Model file for the job. Use its own axes, mm. Face numbers are marked on the shaded views. A direction names the side the tool comes from. Give positions to 0.01 mm unless a question says otherwise; leave off trailing zeros. Write each loop counter-clockwise with the first axis right and the second up, starting at its lowest first coordinate (ties: lowest second). Pieces come first, ordered by that corner, then holes. Notation, with made-up numbers: (28, 67.5) - (67, 67.5) arc R14 cw to (67, 93.5) - close; hole circle Ø9 at (43.25, -29.5). An arc over 180 degrees is marked (long way). Use a Markdown table: item, result. Add a question column.
```python
from build123d import *

# Parameters (mm, degrees)
F2_DEPTH = 35


with BuildPart() as f2:
    # F1 (on Top) + F0 (on Top) → F2 (new body)
    with BuildSketch(Plane.XY):
        Polygon((-16.83088, -2.557084), (0, -2.557084), (0, 0), (-14.142136, 14.142136), (-12.975409, 15.308862), (-10.107344, 12.440796), (-8.69313, 13.85501), (-12.823902, 17.985781), (-14.238115, 16.571568), (-16.83088, 14.142136), align=None)
        Polygon((-14.142136, 11.453391), (-2.688745, 0), (-14.142136, 0), align=None, mode=Mode.SUBTRACT)
    with BuildSketch(Plane.XY):
        Polygon((14.142136, 14.142136), (0, 0), (0, -2.557084), (16.83088, -2.557084), (16.83088, 14.142136), (14.238115, 16.571568), (12.823902, 17.985781), (8.69313, 13.85501), (10.107344, 12.440796), (12.975409, 15.308862), align=None)
        Polygon((2.688745, 0), (14.142136, 11.453391), (14.142136, 0), align=None, mode=Mode.SUBTRACT)
    extrude(amount=F2_DEPTH)


solid = f2.part
```
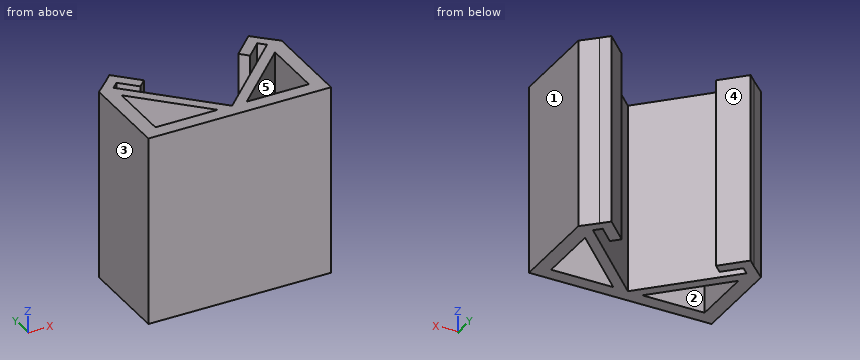
(1) Band-saw the part on C-C (y = 9). Write the cut outline in (x, z).
(2) Band-saw the part on D-D (y = 14.75). Write the cut outline in (x, z).
(3) Probe probe 1 along X at (y, z) = (10, 27); probe 2 along X at (y, z) = (1, 32.5); probe 3 along Y at (x, z) = (13, 11). List the from-to ranges inside material, lowest first. Write a range as [from, to].
(4) Band-saw the part on A-A (z = 11). Write the cut outline in (x, y) (3 decimals).
(5) Two-plate mould, pull along Y, no slides. Class the marked faces 3, 4 and 5: +Y half, -Y half, draft (parallel to the pull), parting line (faces both ways), or undercut.
(6) Which spindle directions (+Z, -Z, +X, -X, +Y, -Y) get a long thin tool onto all of the face, cutting with end or side? Do the marked faces 1 and 2. Say none if no direction does.
(7) Flat gauge pins, fed straight in: pin 1 (1.5 mm diameter, centred on x = 10, y = 2, fed in from +Z); pin 2 (2 mm diameter, centred on x = -11, z = 26.5, fed in from +Y). Where does each tip first touch, or does it go through?
(8) Band-saw the part on B-B (x = -5.5). Write the cut outline in (y, z).
Model answer:
| question | item | result |
|---|---|---|
| 1 | outline | (-16.83, 0) - (-14.14, 0) - (-14.14, 35) - (-16.83, 35) - close; (-11.69, 0) - (-9, 0) - (-9, 35) - (-11.69, 35) - close; (9, 0) - (11.69, 0) - (11.69, 35) - (9, 35) - close; (14.14, 0) - (16.83, 0) - (16.83, 35) - (14.14, 35) - close |
| 2 | outline | (-16.18, 0) - (-13.53, 0) - (-13.53, 35) - (-16.18, 35) - close; (-12.42, 0) - (-9.59, 0) - (-9.59, 35) - (-12.42, 35) - close; (9.59, 0) - (12.42, 0) - (12.42, 35) - (9.59, 35) - close; (13.53, 0) - (16.18, 0) - (16.18, 35) - (13.53, 35) - close |
| 3 | probe 1 | x = [-16.83, -14.14], [-12.69, -10], [10, 12.69], [14.14, 16.83] |
| 3 | probe 2 | x = [-16.83, -14.14], [-3.69, -1], [1, 3.69], [14.14, 16.83] |
| 3 | probe 3 | y = [-2.56, 0], [10.31, 13], [15.28, 17.81] |
| 4 | outline | (-16.831, -2.557) - (16.831, -2.557) - (16.831, 14.142) - (14.238, 16.572) - (12.824, 17.986) - (8.693, 13.855) - (10.107, 12.441) - (12.975, 15.309) - (14.142, 14.142) - (0, 0) - (-14.142, 14.142) - (-12.975, 15.309) - (-10.107, 12.441) - (-8.693, 13.855) - (-12.824, 17.986) - (-14.238, 16.572) - (-16.831, 14.142) - close; hole (-14.142, 0) - (-2.689, 0) - (-14.142, 11.453) - close; hole (2.689, 0) - (14.142, 0) - (14.142, 11.453) - close |
| 5 | face 3 | draft |
| 5 | face 4 | +Y half |
| 5 | face 5 | undercut |
| 6 | face 1 | +Z, -Z, +X, +Y, -Y |
| 6 | face 2 | +Z, -Z |
| 7 | pin 1 | passes through |
| 7 | pin 2 | stops at y = 17.16 |
| 8 | outline | (-2.56, 0) - (0, 0) - (0, 35) - (-2.56, 35) - close; (2.81, 0) - (5.5, 0) - (5.5, 35) - (2.81, 35) - close |
